Here's how the part is built. I have some questions about the finished solid (model axes, mm). Face numbers are marked on the shaded views. A direction names the side the tool comes from. Coordinates: 2 decimals unless noted, no trailing zeros. Loops run counter-clockwise (first coordinate to the right, second up) from the corner with the lowest first, then second, coordinate; pieces in that order, holes last. Notation, with made-up numbers: (-21.75, 86.5) -> (25.25, 86.5) arc R23 ccw to (25.25, 119.5) -> close; hole circle Ø9 at (-30.75, -8). An arc over 180 degrees is marked (long way). Answer as a JSON object with one key per item and string values. Group by question number.
1) If we mould it in two halves opening along Y, with no side actions, what happens to the marked faces 1, 2 and 3? For each: +Y half, -Y half, draft (parallel to the pull), parting line (faces both ways), or undercut.
2) I need wall thicknesses on probe 1 along X at (y, z) = (6.25, 11.5); probe 2 along Z at (x, y) = (-8.25, 0). Which ranges of each line are inside material? Lowest first, please. Write a range as [from, to].
3) I want a section at A-A (y = 0). Count the separate pieces of the cut face and the enclosed holes in it, then the cut area to 3 significant figures.
4) I want a section at B-B (x = -2.5). Write out the boundary of the cut face in (y, z), then the cut area to 3 significant figures.
5) I'm going to push flat-ended pins straight in: pin 1 (2.5 mm diameter, centred on y = 1.5, z = 11.5, fed in from +X); pin 2 (4.5 mm diameter, centred on y = 0, z = 12.5, fed in from -X); pin 3 (0.9 mm diameter, centred on x = -5, y = -1, fed in from +Z); pin 4 (0.8 mm diameter, centred on x = 0.5, y = 1, fed in from +Z). Where does each tip first touch, or does it pass through?
6) Which directions (+Z, -Z, +X, -X, +Y, -Y) give clear straight access to the entire face, cutting with the end or side of a thin tool? Please do the marked faces 4, 5 and 6.
```python
from build123d import *

# Parameters (mm, degrees)
F0_W      = 15
F0_H      = 3
F1_DEPTH  = 15
F2_DEPTH  = 3
F3_DEPTH  = 3
F4_DEPTH  = 2
F5_DEPTH  = 3
F6_DEPTH  = 12
F7_D      = 5
F7_DEPTH  = 15
F9_W      = 3.15
F9_H      = 15
F10_DEPTH = 17
F11_R     = 1


with BuildPart() as f1:
    # F0 (on Right) → F1 (new body)
    with BuildSketch(Plane.YZ):
        with Locations((0, 1.5)):
            Rectangle(F0_W, F0_H)
    extrude(amount=-F1_DEPTH)

    # F0 (on Right) → F2 (join)
    with BuildSketch(Plane.YZ):
        with BuildLine():
            Line((-7.5, 12.5), (-7.5, 3))
            Line((-7.5, 3), (7.5, 3))
            Line((7.5, 3), (7.5, 12.5))
            ThreePointArc((7.5, 12.5), (0, 20), (-7.5, 12.5))
        make_face()
        Polygon((-6.25, 12.5), (-3.125, 17.912659), (3.125, 17.912659), (6.25, 12.5), (3.125, 7.087341), (-3.125, 7.087341), align=None, mode=Mode.SUBTRACT)
    extrude(amount=-F2_DEPTH)

    # F0 (on Right) → F3 (join)
    with BuildSketch(Plane.YZ):
        Polygon((3.125, 17.912659), (-3.125, 17.912659), (-6.25, 12.5), (-3.125, 7.087341), (3.125, 7.087341), (6.25, 12.5), align=None)
        Polygon((-4.907477, 12.5), (-2.453739, 16.75), (2.453739, 16.75), (4.907477, 12.5), (2.453739, 8.25), (-2.453739, 8.25), align=None, mode=Mode.SUBTRACT)
    extrude(amount=-F3_DEPTH)

    # F0 (on Right) → F4 (join)
    with BuildSketch(Plane.YZ):
        Polygon((3.125, 17.912659), (-3.125, 17.912659), (-6.25, 12.5), (-3.125, 7.087341), (3.125, 7.087341), (6.25, 12.5), align=None)
        Polygon((-4.907477, 12.5), (-2.453739, 16.75), (2.453739, 16.75), (4.907477, 12.5), (2.453739, 8.25), (-2.453739, 8.25), align=None, mode=Mode.SUBTRACT)
    extrude(amount=F4_DEPTH)

    # F0 (on Right) → F5 (join)
    with BuildSketch(Plane.YZ):
        Polygon((2.453739, 16.75), (-2.453739, 16.75), (-4.907477, 12.5), (-2.453739, 8.25), (2.453739, 8.25), (4.907477, 12.5), align=None)
    extrude(amount=-F5_DEPTH)

    # F5_face (on face) → F6 (join)
    with BuildSketch(Plane(origin=(-3, 0, 10.786279), x_dir=(0, 1, 0), z_dir=(-1, 0, 0))):
        with BuildLine():
            Line((-7.5, 7.786279), (-7.5, -1.713721))
            ThreePointArc((-7.5, -1.713721), (0, -9.213721), (7.5, -1.713721))
            Line((7.5, -1.713721), (7.5, 7.786279))
            Line((7.5, 7.786279), (-7.5, 7.786279))
        make_face()
    extrude(amount=F6_DEPTH)

    # F7
    with Locations(Plane.YZ):
        with Locations((0, 12.5)):
            Hole(F7_D / 2, depth=F7_DEPTH)

    # F9 (on offset) → F10 (cut)
    with BuildSketch(Plane.XY.offset(20)):
        with Locations((-10.475, 0)):
            Rectangle(F9_W, F9_H)
        with Locations((-4.525, 0)):
            Rectangle(F9_W, F9_H)
    extrude(amount=-F10_DEPTH, mode=Mode.SUBTRACT)

    # F11
    f11_edges = [f1.edges().sort_by_distance(p)[0] for p in [
        (2, -4.6875, 9.793671),
        (2, 0, 7.087341),
        (2, -4.6875, 15.206329),
        (2, 0, 17.912659),
        (2, 4.6875, 15.206329),
        (2, 4.6875, 9.793671),
    ]]
    fillet(f11_edges, radius=F11_R)


solid = f1.part
```
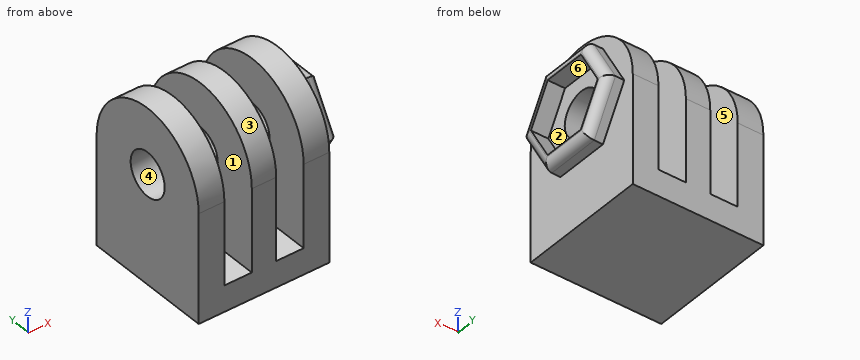
Determined:
{
 "1": {"face 1": "draft", "face 2": "undercut", "face 3": "parting line"},
 "2": {"probe 1": "[-15, -12.05], [-8.9, -6.1], [-2.95, 0]", "probe 2": "[0, 10], [15, 20]"},
 "3": {"separate pieces": "4", "enclosed holes": "0", "area": "154 mm^2"},
 "4": {"outline": "(-7.5, 0) -> (7.5, 0) -> (7.5, 12.5) arc R7.5 ccw to (-7.5, 12.5) -> close; hole circle Ø5 at (0, 12.5)", "area": "256 mm^2"},
 "5": {"pin 1": "x = 0", "pin 2": "through", "pin 3": "z = 3", "pin 4": "z = 17.91"},
 "6": {"face 4": "+X, -X", "face 5": "+Z, +Y, -Y", "face 6": "+X"}
}
